Study the drawing (mm; zero at the part's minimum x, y, z) and answer. A direction names the side the tool comes from. Round coordinates to 2 decimals unless told otherwise and drop trailing zeros. Loops run counter-clockwise (first coordinate to the right, second up) from the corner with the lowest first, then second, coordinate; pieces in that order, holes last. Notation, with made-up numbers: (19, 73) -> (54, 73) arc R25 ccw to (54, 102) -> close; hole circle Ø2 at (61, 3.5). An arc over 180 degrees is marked (long way). Use one line per item in the form item = value.
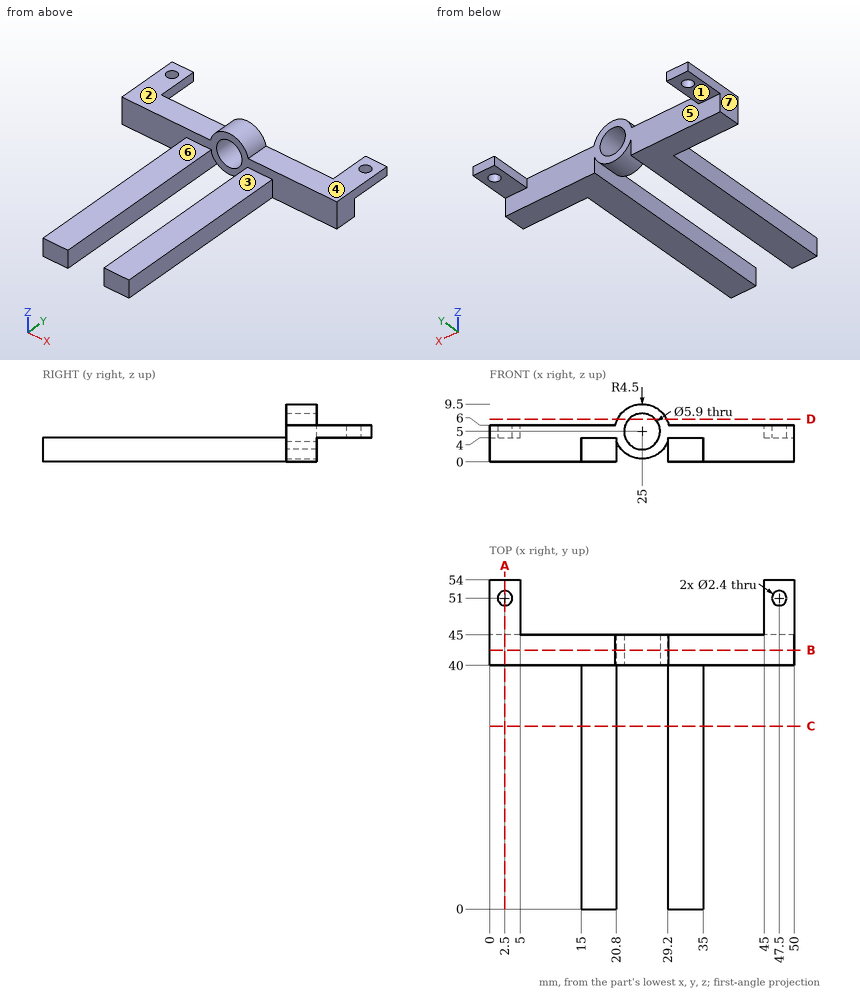
(1) Find section C-C, the plane y = 30. Write down the section's boundary in (x, z).
Completed:
outline = (15, 0) -> (20.8, 0) -> (20.8, 4) -> (15, 4) -> close; (29.2, 0) -> (35, 0) -> (35, 4) -> (29.2, 4) -> close
(2) Find section D-D, the plane z = 7. Write down the section's boundary in (x, y), then the cut area to 3 significant figures.
Completed:
outline = (20.97, 40) -> (22.83, 40) -> (22.83, 45) -> (20.97, 45) -> close; (27.17, 40) -> (29.03, 40) -> (29.03, 45) -> (27.17, 45) -> close
area = 18.6 mm2
(3) For the marked faces 1, 2, 3 and 4, determine the directions among +Z, -Z, +X, -X, +Y, -Y from which every point of the face is accessible in a straight line to the end or side of a thin tool.
Completed:
face_1 = -Z, +X, -X, +Y
face_2 = +Z, -X, +Y, -Y
face_3 = +Z, +X, -X, -Y
face_4 = +Z, +X, +Y, -Y
(4) Given P1, Ø4.5, axis at y = 31, z = 2.5, coming from the +X side; P2, Ø3, axis at x = 32, y = 24.5, coming from the +Z side; P3, Ø1.2, axis at y = 18, z = 3, coming from the -X side; P4, Ø1.9, axis at x = 2.5, y = 51, coming from the -Z side, each flat-ended and moving along its own axis, determine where each tip first touches the part or whether it passes through.
Completed:
P1 = 35
P2 = 4
P3 = 15
P4 = through
(5) Consider L1, parallel to X at y = 51, z = 5.5; L2, parallel to X at y = 2, z = 1.25; L3, parallel to X at y = 41.95, z = 5. Determine where each line is inside the solid, lowest interval first.
Completed:
L1 = 0 to 1.3, 3.7 to 5, 45 to 46.3, 48.7 to 50
L2 = 15 to 20.8, 29.2 to 35
L3 = 0 to 22.05, 27.95 to 50
(6) Find section A-A, the plane x = 2.5. Write down the section's boundary in (y, z), then the cut area to 3 significant figures.
Completed:
outline = (40, 0) -> (45, 0) -> (45, 4) -> (49.8, 4) -> (49.8, 6) -> (40, 6) -> close; (52.2, 4) -> (54, 4) -> (54, 6) -> (52.2, 6) -> close
area = 43.2 mm2
(7) Find section B-B, the plane y = 42.5. Write down the section's boundary in (x, z).
Completed:
outline = (0, 0) -> (20.8, 0) -> (20.8, 3.38) arc R4.5 ccw to (29.2, 3.38) -> (29.2, 0) -> (50, 0) -> (50, 6) -> (29.39, 6) arc R4.5 ccw to (20.61, 6) -> (0, 6) -> close; hole circle Ø5.9 at (25, 5)
(8) For a pull along X with two mould halves and no side action, classify the marked faces 5, 6 and 7 as +X half, -X half, draft (parallel to the pull), parting line (faces both ways), or undercut.
Completed:
face_5 = undercut
face_6 = draft
face_7 = -X half
